from build123d import *

# Parameters (mm, degrees)
SKETCH1_W           = 56
SKETCH1_H           = 90
BOSS_EXTRUDE1_DEPTH = 7
SKETCH2_R           = 14.275
CUT_EXTRUDE1_DEPTH  = 8
CUT_EXTRUDE2_DEPTH  = 8


with BuildPart() as part:
    # Sketch1 → Boss-Extrude1 (new body)
    with BuildSketch(Plane(origin=(0, 0, 0), x_dir=(0, 0, -1), z_dir=(1, 0, 0))):
        with Locations((28, 45)):
            Rectangle(SKETCH1_W, SKETCH1_H)
    extrude(amount=BOSS_EXTRUDE1_DEPTH)

    # Sketch2 → Cut-Extrude1 (cut, through all)
    with BuildSketch(Plane(origin=(7, 0, 0), x_dir=(0, 0, -1), z_dir=(1, 0, 0))):
        with Locations((28, 21.516289278)):
            Circle(SKETCH2_R)
    extrude(amount=-CUT_EXTRUDE1_DEPTH, mode=Mode.SUBTRACT)

    # Sketch3 → Cut-Extrude2 (cut, through all)
    with BuildSketch(Plane(origin=(7, 0, 0), x_dir=(0, 0, -1), z_dir=(1, 0, 0))):
        with BuildLine():
            Line((10.25, 71.244817418), (10.25, 8.434985259))
            ThreePointArc((10.25, 8.434985259), (7.5, 5.684985259), (4.75, 8.434985259))
            Line((4.75, 8.434985259), (4.75, 71.244817418))
            ThreePointArc((4.75, 71.244817418), (7.5, 73.994817418), (10.25, 71.244817418))
        make_face()
        with BuildLine():
            Line((45.75, 8.434985259), (45.75, 71.244817418))
            ThreePointArc((45.75, 71.244817418), (48.5, 73.994817418), (51.25, 71.244817418))
            Line((51.25, 71.244817418), (51.25, 8.434985259))
            ThreePointArc((51.25, 8.434985259), (48.5, 5.684985259), (45.75, 8.434985259))
        make_face()
    extrude(amount=-CUT_EXTRUDE2_DEPTH, mode=Mode.SUBTRACT)


solid = part.part
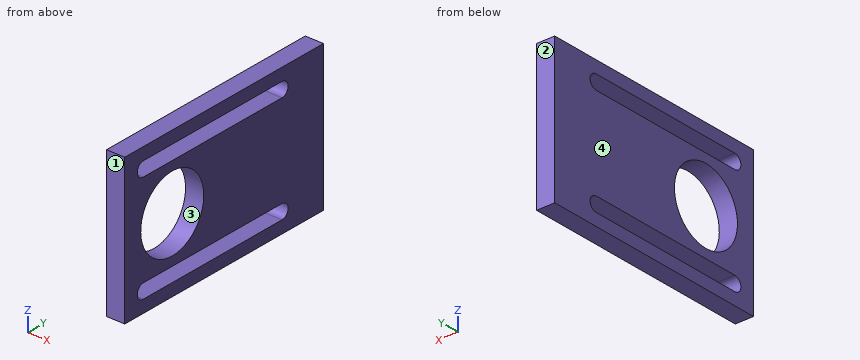
Input: part model. Units: mm. Frame: model coordinates. Face numbers are marked on the shaded views. Give positions to 0.01 mm unless a question says otherwise; leave off trailing zeros. Loops run counter-clockwise (first coordinate to the right, second up) from the corner with the lowest first, then second, coordinate; pieces in that order, holes last. Notation, with made-up numbers: M -26.5,80 L -14.5,80 A24 cw -14.5,119 Z; hole C 47,56 d4. An arc over 180 degrees is marked long. Use one line per item in the form item = value.
1. Section query A-A, the plane z = -7.5. Return the cut outline in (x, y).
Numbers:
outline = M 0,0 L 7,0 L 7,5.68 L 0,5.68 Z; M 0,73.99 L 7,73.99 L 7,90 L 0,90 Z
2. Line query: L1, parallel to Z at x = 4.25, y = 54; L2, parallel to Y at x = 2.5, z = -28; L3, parallel to Z at x = 1.5, y = 18.5. Output: solid intervals per line, ascending.
Numbers:
L1 = -56 to -51.25, -45.75 to -10.25, -4.75 to 0
L2 = 0 to 7.24, 35.79 to 90
L3 = -56 to -51.25, -45.75 to -41.95, -14.05 to -10.25, -4.75 to 0
3. Section query B-B, the plane y = 63. Return the cut outline in (x, z), and give its area (3 significant figures).
Numbers:
outline = M 0,-56 L 7,-56 L 7,-51.25 L 0,-51.25 Z; M 0,-45.75 L 7,-45.75 L 7,-10.25 L 0,-10.25 Z; M 0,-4.75 L 7,-4.75 L 7,0 L 0,0 Z
area = 315 mm²
4. Section query D-D, the plane z = -28. Return the cut outline in (x, y).
Numbers:
outline = M 0,0 L 7,0 L 7,7.24 L 0,7.24 Z; M 0,35.79 L 7,35.79 L 7,90 L 0,90 Z
5. Section query C-C, the plane x = 5.5. Return the cut outline in (y, z) (3 decimals).
Numbers:
outline = M 0,-56 L 90,-56 L 90,0 L 0,0 Z; hole C 21.516,-28 d28.55; hole M 8.435,-51.25 L 71.245,-51.25 A2.75 ccw 71.245,-45.75 L 8.435,-45.75 A2.75 ccw Z; hole M 8.435,-10.25 L 71.245,-10.25 A2.75 ccw 71.245,-4.75 L 8.435,-4.75 A2.75 ccw Z
6. Pull-direction query (Y, two-part tool) for the marked faces 1, 2, 3 and 4; classes: released by +Y, released by -Y, zero draft, split by the parting line, or undercut.
Numbers:
face_1 = released by -Y
face_2 = released by +Y
face_3 = undercut
face_4 = zero draft
